Design review of the part built by this model. Coordinates are the model's own, in mm. Face numbers are marked on the shaded views. Round coordinates to 2 decimals unless told otherwise and drop trailing zeros. Loops run counter-clockwise (first coordinate to the right, second up) from the corner with the lowest first, then second, coordinate; pieces in that order, holes last. Notation, with made-up numbers: M -16.5,81.25 L 13.5,81.25 A9 ccw 13.5,88.25 Z; hole C -0.75,-17.75 d11. An arc over 180 degrees is marked long. One line per item, written item: value. Start each with the question number.
Item 1: We need section D-D (y = 34). Write out the cut boundary in (x, z) (3 decimals), then the cut area to 3 significant figures.
Item 2: For line 1 along Z through (x, y) = (0, 7.8) (3 decimals); line 2 along X through (y, z) = (42.85, 0) (3 decimals); line 3 along X through (y, z) = (4.35, 0) (3 decimals), list the stretches that pass through material, from the lowest coordinate up.
Item 3: Mouldability with a two-part tool opening along X and no side actions: class the marked faces 1, 2 and 3 as released by +X, released by -X, zero draft, split by the parting line, or undercut.
Item 4: We need section A-A (z = 0). Write out the cut boundary in (x, y) (3 decimals).
Item 5: We need section C-C (x = 3.75). Write out the cut boundary in (y, z) (3 decimals), then the cut area to 3 significant figures.
Item 6: We need section B-B (y = 12). Write out the cut boundary in (x, z) (3 decimals), then the cut area to 3 significant figures.
Item 7: Clearance check with flat-ended pins moving along their axes: pin 1 (5 mm diameter, centred on x = -3, z = -2.5, fed in from -Y); pin 2 (7 mm diameter, centred on x = -1.5, y = 22, fed in from -Z) (3 decimals); pin 3 (4 mm diameter, centred on x = -2.5, y = 12.5, fed in from +Z). State where each tip first meets the part, or that it passes through.
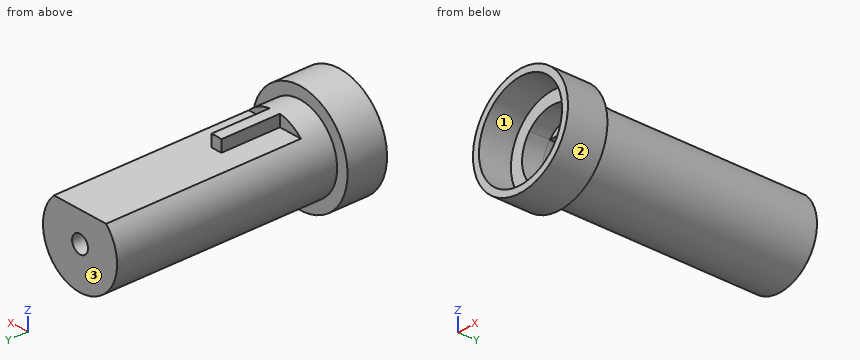
from build123d import *

# Parameters (mm, degrees)
SKETCH1_R           = 9.005
BASE_RING_DEPTH     = 6.69
SKETCH2_R           = 7.025
MAIN_CYLINDER_DEPTH = 44
CUTOUT_PT1_DEPTH    = 33.03
CUTOUT_PT2_DEPTH    = 23.11
SKETCH5_R           = 1.505
TOP_HOLE_DEPTH      = 46.805895363
SKETCH7_R           = 7.875
CUT_EXTRUDE4_DEPTH  = 5.42
SKETCH8_R           = 5.76
CUT_EXTRUDE5_DEPTH  = 8.86
CUT_EXTRUDE6_DEPTH  = 40.88


with BuildPart() as part:
    # Sketch1 → Base Ring (new body)
    with BuildSketch(Plane(origin=(0, 0, 0), x_dir=(1, 0, 0), z_dir=(0, 1, 0))):
        with Locations(Location((0, 0, 0), (0, 0, 270))):
            Circle(SKETCH1_R)
    extrude(amount=BASE_RING_DEPTH)

    # Sketch2 → Main Cylinder (add)
    with BuildSketch(Plane(origin=(0, 0, 0), x_dir=(1, 0, 0), z_dir=(0, 1, 0))):
        with Locations(Location((0, 0, 0), (0, 0, 270))):
            Circle(SKETCH2_R)
    extrude(amount=MAIN_CYLINDER_DEPTH)

    # Sketch3 → Cutout pt1 (cut)
    with BuildSketch(Plane(origin=(0, 44, 0), x_dir=(1, 0, 0), z_dir=(0, 1, 0))):
        with BuildLine():
            Line((-4.939696347, -4.995), (-0.96, -4.995))
            Line((-0.96, -4.995), (-0.96, -6.959096565))
            ThreePointArc((-0.96, -6.959096565), (-3.109022849, -6.299571567), (-4.939696347, -4.995))
        make_face()
        with BuildLine():
            Line((0.96, -4.995), (0.96, -6.959096565))
            ThreePointArc((0.96, -6.959096565), (3.109022849, -6.299571567), (4.939696347, -4.995))
            Line((4.939696347, -4.995), (0.96, -4.995))
        make_face()
    extrude(amount=-CUTOUT_PT1_DEPTH, mode=Mode.SUBTRACT)

    # Sketch4 → Cutout pt2 (cut)
    with BuildSketch(Plane(origin=(0, 44, 0), x_dir=(1, 0, 0), z_dir=(0, 1, 0))):
        with BuildLine():
            Line((-0.96, -4.995), (0.96, -4.995))
            Line((0.96, -4.995), (0.96, -6.959096565))
            ThreePointArc((0.96, -6.959096565), (0, -7.025), (-0.96, -6.959096565))
            Line((-0.96, -6.959096565), (-0.96, -4.995))
        make_face()
    extrude(amount=-CUTOUT_PT2_DEPTH, mode=Mode.SUBTRACT)

    # Sketch5 → Top Hole (cut, through all)
    with BuildSketch(Plane(origin=(0, 44, 0), x_dir=(1, 0, 0), z_dir=(0, 1, 0))):
        with Locations(Location((0, 0, 0), (0, 0, 270))):
            Circle(SKETCH5_R)
    extrude(amount=-TOP_HOLE_DEPTH, mode=Mode.SUBTRACT)

    # Sketch7 → Cut-Extrude4 (cut)
    with BuildSketch(Plane(origin=(0, 0, 0), x_dir=(1, 0, 0), z_dir=(0, 1, 0))):
        with Locations(Location((0, 0, 0), (0, 0, 270))):
            Circle(SKETCH7_R)
    extrude(amount=CUT_EXTRUDE4_DEPTH, mode=Mode.SUBTRACT)

    # Sketch8 → Cut-Extrude5 (cut)
    with BuildSketch(Plane(origin=(0, 0, 0), x_dir=(1, 0, 0), z_dir=(0, 1, 0))):
        with Locations(Location((0, 0, 0), (0, 0, 270))):
            Circle(SKETCH8_R)
    extrude(amount=CUT_EXTRUDE5_DEPTH, mode=Mode.SUBTRACT)

    # Sketch9 → Cut-Extrude6 (cut)
    with BuildSketch(Plane(origin=(0, 0, 0), x_dir=(1, 0, 0), z_dir=(0, 1, 0))):
        with BuildLine():
            Line((4.33745317, -3.79), (-4.33745317, -3.79))
            ThreePointArc((-4.33745317, -3.79), (0, 5.76), (4.33745317, -3.79))
        make_face()
    extrude(amount=CUT_EXTRUDE6_DEPTH, mode=Mode.SUBTRACT)


solid = part.part
A:
1. outline: M -4.94,4.995 A7.025 ccw long 4.94,4.995 Z; hole M -4.337,3.79 A5.76 ccw long 4.337,3.79 Z
1. area: 48.8 mm2
2. line 1: -7.025 to -5.76, 5.76 to 7.025
2. line 2: -7.025 to -1.505, 1.505 to 7.025
2. line 3: -9.005 to -7.875, 7.875 to 9.005
3. face 1: undercut
3. face 2: split by the parting line
3. face 3: zero draft
4. outline: M -9.005,0 L -7.875,0 L -7.875,5.42 L -5.76,5.42 L -5.76,40.88 L -1.505,40.88 L -1.505,44 L -7.025,44 L -7.025,6.69 L -9.005,6.69 Z; M 1.505,40.88 L 5.76,40.88 L 5.76,5.42 L 7.875,5.42 L 7.875,0 L 9.005,0 L 9.005,6.69 L 7.025,6.69 L 7.025,44 L 1.505,44 Z
5. outline: M 0,-8.187 L 6.69,-8.187 L 6.69,-5.94 L 44,-5.94 L 44,4.995 L 10.97,4.995 L 10.97,5.94 L 6.69,5.94 L 6.69,8.187 L 0,8.187 L 0,6.925 L 5.42,6.925 L 5.42,4.372 L 8.86,4.372 L 8.86,3.79 L 40.88,3.79 L 40.88,-4.372 L 5.42,-4.372 L 5.42,-6.925 L 0,-6.925 Z
5. area: 155 mm2
6. outline: M -4.94,4.995 A7.025 ccw long 4.94,4.995 L 0.96,4.995 L 0.96,6.959 A7.025 ccw -0.96,6.959 L -0.96,4.995 Z; hole M -4.337,3.79 A5.76 ccw long 4.337,3.79 Z
6. area: 52.7 mm2
7. pin 1: y = 5.42
7. pin 2: z = -7.025
7. pin 3: z = 7.01
